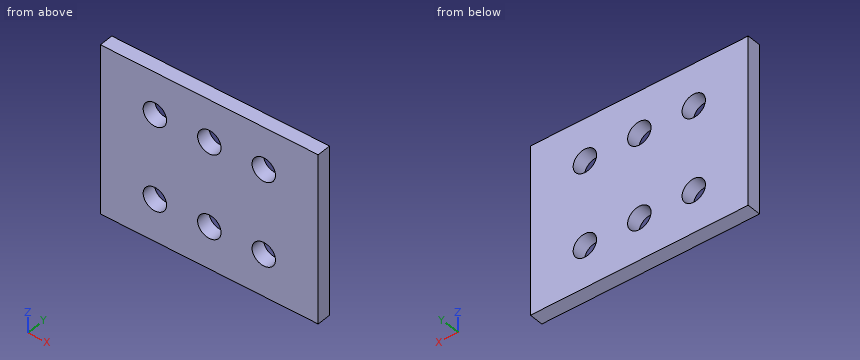
Autodesk Inventor part; units mm, degrees
ref_plane "YZ Plane" through (0, 0, 0) normal (1, 0, 0) x (0, 1, 0)
ref_plane "XZ Plane" through (0, 0, 0) normal (0, 1, 0) x (-1, 0, 0)
ref_plane "XY Plane" through (0, 0, 0) normal (0, 0, 1) x (1, 0, 0)
sketch "Sketch1" plane through (0, 0, 0) normal (0, 1, 0) x (-1, 0, 0)
  line L0 (0, 0) -> (46.5, 0)
  line L1 (46.5, 0) -> (46.5, -36)
  line L2 (46.5, -36) -> (0, -36)
  line L3 (0, -36) -> (0, 0)
  circle A0 centre (34.875, -27) radius 2.5
  circle A1 centre (11.625, -27) radius 2.5
  circle A2 centre (23.25, -27) radius 2.5
  line L4 (46.5, -18) -> (0, -18)
  circle A3 centre (34.875, -9) radius 2.5
  circle A4 centre (11.625, -9) radius 2.5
  circle A5 centre (23.25, -9) radius 2.5
  dimension "d0" = 46.5
  dimension "d1" = 36
  dimension "d2" = 5
  dimension "d3" = 11.625
  dimension "d4" = 27
  dimension "d6" = 5
  dimension "d7" = 11.625
  dimension "d13" = 5
  dimension "d15" = 11.625
extrude "Extrusion6" add sketch "Sketch1" along normal blind 3
properties part number "chassiconnector"
Read the model definition and answer for the solid it produces. Units are mm, in the model's axes. Round coordinates to 2 decimals unless told otherwise and drop trailing zeros. Write each loop counter-clockwise with the first axis right and the second up, starting at its lowest first coordinate (ties: lowest second). Pieces come first, ordered by that corner, then holes.
1. Given pin 1 Ø4.5 at (x, z) = (-23.25, -27) entering from +Y, flat-ended and moving along its own axis, determine where the tip first touches the part or whether it passes through.
2. The part is cut by section B-B, the plane x = -23.25. Determine the outline of the cut face in (y, z).
3. The part is cut by section A-A, the plane z = -9. Determine the outline of the cut face in (x, y) (3 decimals), then the cut area to 3 significant figures.
4. Straight lines are drawn through the part: L1, parallel to Z at x = -35, y = 2.3; L2, parallel to X at y = 0.35, z = -7.5 (3 decimals); L3, parallel to Z at x = -34, y = 1.05. For each, find the intervals that lie inside material, in ascending order.
5. The part is cut by section C-C, the plane y = 2.3. Determine the outline of the cut face in (x, z) (3 decimals).
Values:
1. pin 1: passes through
2. outline: (0, -36) - (3, -36) - (3, -29.5) - (0, -29.5) - close; (0, -24.5) - (3, -24.5) - (3, -11.5) - (0, -11.5) - close; (0, -6.5) - (3, -6.5) - (3, 0) - (0, 0) - close
3. outline: (-46.5, 0) - (-37.375, 0) - (-37.375, 3) - (-46.5, 3) - close; (-32.375, 0) - (-25.75, 0) - (-25.75, 3) - (-32.375, 3) - close; (-20.75, 0) - (-14.125, 0) - (-14.125, 3) - (-20.75, 3) - close; (-9.125, 0) - (0, 0) - (0, 3) - (-9.125, 3) - close
3. area: 94.5 mm2
4. L1: z = -36 to -29.5, -24.5 to -11.5, -6.5 to 0
4. L2: x = -46.5 to -36.875, -32.875 to -25.25, -21.25 to -13.625, -9.625 to 0
4. L3: z = -36 to -29.34, -24.66 to -11.34, -6.66 to 0
5. outline: (-46.5, -36) - (0, -36) - (0, 0) - (-46.5, 0) - close; hole circle Ø5 at (-34.875, -27); hole circle Ø5 at (-34.875, -9); hole circle Ø5 at (-23.25, -27); hole circle Ø5 at (-23.25, -9); hole circle Ø5 at (-11.625, -27); hole circle Ø5 at (-11.625, -9)
